Verification items for the finished model (mm, model axes). A direction names the side the tool comes from. Coordinates: 2 decimals unless noted, no trailing zeros. Loops run counter-clockwise (first coordinate to the right, second up) from the corner with the lowest first, then second, coordinate; pieces in that order, holes last. Notation, with made-up numbers: (59.25, 76.5) - (85.25, 76.5) arc R22 cw to (85.25, 103.5) - close; hole circle Ø3 at (63, 71). An arc over 180 degrees is marked (long way). One line per item, written item: value. Start each with the question number.
(1) Set-up check for faces 1 (the face through (2.2, 3, -1)), 2 (the face through (0, 2, 41)), 3 (the face through (10, 1, -4)): record each of +Z, -Z, +X, -X, +Y, -Y from which the full face is reachable in a straight line by a thin tool's end or side.
(2) Section check D-D (x = 4). Record the boundary of the cut face in (y, z).
(3) Gauge pin test, flat ends, axial feed: P1, Ø1.5, axis at y = 1, z = 40, coming from the +X side; P2, Ø0.9, axis at y = 1.5, z = -4.5, coming from the +X side; P3, Ø5.5, axis at x = 0, z = 62.5, coming from the -Y side; P4, Ø1.5, axis at y = 2, z = -44, coming from the +X side. Record the tip position at first contact, or that the pin passes through.
(4) Section check B-B (x = 50). Record the boundary of the cut face in (y, z).
(5) Section check A-A (z = 62.5). Record the boundary of the cut face in (x, y).
(6) Draft check along Z on faces 4 (the face through (57.5, 1.5, -70)), 5 (the face through (57.5, 1.5, 70)), 6 (the face through (48.137, 1.479, -61.531)). Enter one of: +Z half, -Z half, draft (parallel to the pull), parting line (faces both ways), or undercut.
(7) Thickness scan on probe 1 along X at (y, z) = (1, 62.5); probe 2 along X at (y, z) = (2.15, 0); probe 3 along X at (y, z) = (0.3, -64). Record the ranges inside material, lowest first. Write a range as [from, to].
(8) Section check C-C (z = 0). Record the boundary of the cut face in (x, y).
```python
from build123d import *
from OCP.BRepFilletAPI import BRepFilletAPI_MakeChamfer

# Parameters (mm, degrees)
SKETCH_1_R          = 2.1
EXTRUDE_1_DEPTH     = 3
CHAMFER_1_SIZE      = 5
CHAMFER_1_SIZE2     = 13.660254038
FILLET_1_R          = 3
CUT_EXTRUDE_1_DEPTH = 10
FILLET_2_R          = 1.5


with BuildPart() as part:
    # 草图1 → 凸台-拉伸1 (new body)
    # profile 1 of 3: a face of its own
    with BuildSketch(Plane(origin=(0, 0, 0), x_dir=(1, 0, 0), z_dir=(0, 1, 0))):
        Polygon((10, 52.5), (10, 23.632486541), (60, 52.5), align=None)
    # profile 2 of 3: a face of its own
    with BuildSketch(Plane(origin=(0, 0, 0), x_dir=(1, 0, 0), z_dir=(0, 1, 0))):
        Polygon((10, -23.632486541), (10, -52.5), (60, -52.5), align=None)
    # profile 3 of 3: a face of its own
    with BuildSketch(Plane(origin=(0, 0, 0), x_dir=(1, 0, 0), z_dir=(0, 1, 0))):
        Polygon((60, -52.5), (60, -72.5), (-10, -72.5), (-10, 72.5), (60, 72.5), (60, 52.5), (10, 52.5), (10, -52.5), align=None)
        with Locations(Location((50, -62.5, 0), (0, 0, 270))):
            Circle(SKETCH_1_R, mode=Mode.SUBTRACT)
        with Locations(Location((0, 0, 0), (0, 0, 270))):
            Circle(SKETCH_1_R, mode=Mode.SUBTRACT)
        with Locations(Location((50, 62.5, 0), (0, 0, 270))):
            Circle(SKETCH_1_R, mode=Mode.SUBTRACT)
        with Locations(Location((0, 62.5, 0), (0, 0, 270))):
            Circle(SKETCH_1_R, mode=Mode.SUBTRACT)
        with Locations(Location((0, -62.5, 0), (0, 0, 270))):
            Circle(SKETCH_1_R, mode=Mode.SUBTRACT)
    extrude(amount=EXTRUDE_1_DEPTH)

    # 倒角1: one chamfer whose edges measure the first distance from different faces: ONE call of the kernel's chamfer builder (chamfer() names one face for all edges)
    chamfer_1_edges_1 = [part.edges().sort_by_distance(p)[0] for p in [
        (60, 1.5, 72.5),
        (-10, 1.5, 72.5),
        (-10, 1.5, -72.5),
        (60, 1.5, -72.5),
    ]]
    chamfer_1_edges_2 = [part.edges().sort_by_distance(p)[0] for p in [
        (10, 1.5, -23.632486541),
    ]]
    chamfer_1_side_2 = [part.faces().sort_by_distance(p)[0] for p in [
        (10, 1.5, 0),
    ]]
    chamfer_1_edges_3 = [part.edges().sort_by_distance(p)[0] for p in [
        (10, 1.5, 23.632486541),
    ]]
    chamfer_1_side_3 = [part.faces().sort_by_distance(p)[0] for p in [
        (35, 1.5, 38.06624327),
    ]]
    chamfer_1 = BRepFilletAPI_MakeChamfer(part.part.solid().wrapped)
    for e in chamfer_1_edges_1:
        chamfer_1.Add(CHAMFER_1_SIZE, e.wrapped)
    for e in chamfer_1_edges_2:
        chamfer_1.Add(CHAMFER_1_SIZE, CHAMFER_1_SIZE2, e.wrapped, chamfer_1_side_2[0].wrapped)  # the first distance lies on this face
    for e in chamfer_1_edges_3:
        chamfer_1.Add(CHAMFER_1_SIZE, CHAMFER_1_SIZE2, e.wrapped, chamfer_1_side_3[0].wrapped)  # the first distance lies on this face
    add(Compound.cast(chamfer_1.Shape()), mode=Mode.REPLACE)

    # 圆角1
    fillet_1_edges = [part.edges().sort_by_distance(p)[0] for p in [
        (60, 1.5, -52.5),
        (60, 1.5, 52.5),
        (60, 1.5, 67.5),
        (-5, 1.5, 72.5),
        (55, 1.5, 72.5),
        (-10, 1.5, -67.5),
        (-10, 1.5, 67.5),
        (10, 1.5, -18.632486541),
        (10, 1.5, 9.972232503),
        (14.330127019, 1.5, 26.132486541),
        (21.830127019, 1.5, -30.462613559),
        (-5, 1.5, -72.5),
        (55, 1.5, -72.5),
        (60, 1.5, -67.5),
    ]]
    fillet(fillet_1_edges, radius=FILLET_1_R)

    # 草图3 → 切除-拉伸1 (cut)
    with BuildSketch(Plane(origin=(0, 3, 0), x_dir=(1, 0, 0), z_dir=(0, 1, 0))):
        Polygon((0, -52.5), (0, -29.126059631), (50, -52.5), align=None)
        Polygon((0, 52.5), (0, 29.126059631), (50, 52.5), align=None)
    extrude(amount=-CUT_EXTRUDE_1_DEPTH, mode=Mode.SUBTRACT)

    # 圆角2
    fillet_2_edges = [part.edges().sort_by_distance(p)[0] for p in [
        (0, 1.5, 52.5),
        (0, 1.5, 29.126059631),
        (50, 1.5, 52.5),
        (0, 1.5, -52.5),
        (50, 1.5, -52.5),
        (0, 1.5, -29.126059631),
    ]]
    fillet(fillet_2_edges, radius=FILLET_2_R)


solid = part.part
```
Responses:
1. face 1: +Z, -Z, +X, -X, +Y
1. face 2: +Y, -Y
1. face 3: +X, +Y, -Y
2. outline: (0, -72.5) - (3, -72.5) - (3, -52.5) - (0, -52.5) - close; (0, -31) - (3, -31) - (3, 31) - (0, 31) - close; (0, 52.5) - (3, 52.5) - (3, 72.5) - (0, 72.5) - close
3. P1: stops at x = 39.65
3. P2: stops at x = 10
3. P3: stops at y = 0
3. P4: stops at x = 46.58
4. outline: (0, -72.5) - (3, -72.5) - (3, -64.6) - (0, -64.6) - close; (0, -60.4) - (3, -60.4) - (3, -46.73) - (0, -46.73) - close; (0, 46.73) - (3, 46.73) - (3, 60.4) - (0, 60.4) - close; (0, 64.6) - (3, 64.6) - (3, 72.5) - (0, 72.5) - close
5. outline: (-10, 0) - (-2.1, 0) - (-2.1, 3) - (-10, 3) - close; (2.1, 0) - (47.9, 0) - (47.9, 3) - (2.1, 3) - close; (52.1, 0) - (60, 0) - (60, 3) - (52.1, 3) - close
6. face 4: -Z half
6. face 5: +Z half
6. face 6: undercut
7. probe 1: x = [-10, -2.1], [2.1, 47.9], [52.1, 60]
7. probe 2: x = [-10, -2.1], [2.1, 10]
7. probe 3: x = [-10, -1.47], [1.47, 48.53], [51.47, 60]
8. outline: (-10, 0) - (-2.1, 0) - (-2.1, 3) - (-10, 3) - close; (2.1, 0) - (10, 0) - (10, 3) - (2.1, 3) - close
